from build123d import *

# Parameters (mm, degrees)
EXTRUDE_THIN1_DEPTH = 150
FILLET1_R           = 0.1


with BuildPart() as part:
    # Sketch1 → Extrude-Thin1 (new, symmetric)
    with BuildSketch(Plane.XY):
        with BuildLine():
            Line((14.416629547, 0), (14.416629547, 0.55))
            Line((14.416629547, 0.55), (15.440207252, 0.55))
            ThreePointArc((15.440207252, 0.55), (10.924799769, 10.924799769), (0.55, 15.440207252))
            Line((0.55, 15.440207252), (0.55, 14.416629547))
            Line((0.55, 14.416629547), (0, 14.416629547))
            Line((0, 14.416629547), (0, 13.516629547))
            Line((0, 13.516629547), (1.45, 13.516629547))
            Line((1.45, 13.516629547), (1.45, 14.477568857))
            ThreePointArc((1.45, 14.477568857), (10.288403666, 10.288403666), (14.477568857, 1.45))
            Line((14.477568857, 1.45), (13.516629547, 1.45))
            Line((13.516629547, 1.45), (13.516629547, 0))
            Line((13.516629547, 0), (14.416629547, 0))
        make_face()
    extrude(amount=EXTRUDE_THIN1_DEPTH, both=True)

    # Fillet1
    fillet1_edges = [part.edges().sort_by_distance(p)[0] for p in [
        (13.516629547, 1.45, 0),
        (14.477568857, 1.45, 0),
        (1.45, 14.477568857, 0),
        (1.45, 13.516629547, 0),
        (0, 13.516629547, 0),
        (0, 14.416629547, 0),
        (0.55, 14.416629547, 0),
        (0.55, 15.440207252, 0),
        (15.440207252, 0.55, 0),
        (14.416629547, 0.55, 0),
        (14.416629547, 0, 0),
        (13.516629547, 0, 0),
    ]]
    fillet(fillet1_edges, radius=FILLET1_R)


solid = part.part
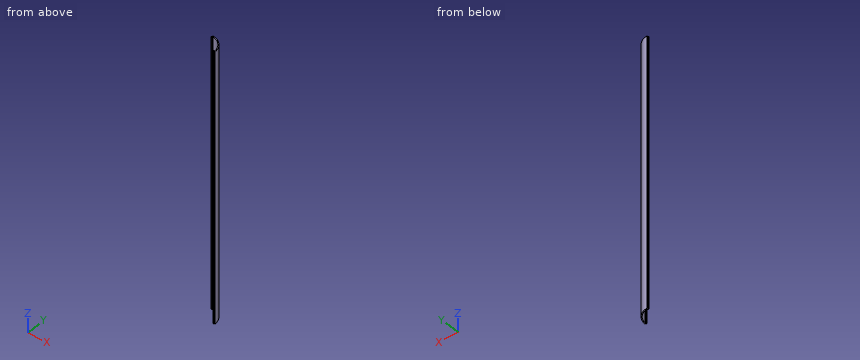
Geometry check sheet. Reference: the model listing, model coordinates, mm. Give positions to 0.01 mm unless a question says otherwise; leave off trailing zeros. Write each loop counter-clockwise with the first axis right and the second up, starting at its lowest first coordinate (ties: lowest second). Pieces come first, ordered by that corner, then holes. Notation, with made-up numbers: (43.5, 46.5) - (49.5, 46.5) arc R24 cw to (49.5, 63.5) - close; hole circle Ø11 at (2, 54). An arc over 180 degrees is marked (long way). Put each result on its own line as item: value.
1. Thickness scan on line 1 (X direction, y = 2, z = 102); line 2 (Y direction, x = 0.5, z = 66); line 3 (X direction, y = 11.5, z = 8.5). Record the ranges inside material, lowest first.
Ans:
line 1: x = 14.41 to 15.32
line 2: y = 13.52 to 14.43
line 3: x = 8.91 to 10.32
2. Go/stop test with flat-tipped pins: pin 1 (0.7 mm diameter, centred on y = 15, z = -9.5, fed in from -X); pin 2 (2 mm diameter, centred on x = 9.5, z = -9, fed in from -Y); pin 3 (6 mm diameter, centred on x = 2.5, z = -82, fed in from +Y); pin 4 (6 mm diameter, centred on y = 5.5, z = 56.5, fed in from -X). Record where each tip stops, or that it passes through.
Ans:
pin 1: stops at x = 0.55
pin 2: stops at y = 10.07
pin 3: stops at y = 15.44
pin 4: stops at x = 11.81
3. Sectioned sample at C-C, the plane x = 11. Enter the section's corners in (y, z), plus the area to 3 significant figures.
Ans:
outline: (9.52, -150) - (10.85, -150) - (10.85, 150) - (9.52, 150) - close
area: 398 mm²
4. Sectioned sample at A-A, the plane z = -97. Enter the section's corners in (x, y).
Ans:
outline: (0, 13.62) arc R0.1 ccw to (0.1, 13.52) - (1.35, 13.52) arc R0.1 ccw to (1.45, 13.62) - (1.45, 14.37) arc R0.1 cw to (1.56, 14.47) arc R14.55 cw to (14.47, 1.56) arc R0.1 cw to (14.37, 1.45) - (13.62, 1.45) arc R0.1 ccw to (13.52, 1.35) - (13.52, 0.1) arc R0.1 ccw to (13.62, 0) - (14.32, 0) arc R0.1 ccw to (14.42, 0.1) - (14.42, 0.45) arc R0.1 cw to (14.52, 0.55) - (15.34, 0.55) arc R0.1 ccw to (15.44, 0.65) arc R15.45 ccw to (0.65, 15.44) arc R0.1 ccw to (0.55, 15.34) - (0.55, 14.52) arc R0.1 cw to (0.45, 14.42) - (0.1, 14.42) arc R0.1 ccw to (0, 14.32) - close
5. Sectioned sample at B-B, the plane y = 6. Enter the section's corners in (x, z).
Ans:
outline: (13.26, -150) - (14.24, -150) - (14.24, 150) - (13.26, 150) - close
